Read the model definition and answer for the solid it produces. Units are mm, in the model's axes. A direction names the side the tool comes from. Coordinates: 2 decimals unless noted, no trailing zeros. Order: outer loops, then holes, each group sorted by start corner. A loop starts at its lowest first (then second) coordinate and runs counter-clockwise, first axis right, second up. Notation, with made-up numbers: (-29.75, 88) - (-14.75, 88) arc R8 ccw to (-14.75, 93) - close; hole circle Ø7 at (-9, 14). An arc over 180 degrees is marked (long way). Use one line per item in the form item = value. Start each with the question number.
from build123d import *

# Parameters (mm, degrees)
RESSALTO_EXTRUS_O1_DEPTH     = 181.5
CORTE_EXTRUS_O2_DEPTH        = 50
FURO_DE_DI_METRO_5_5_5_5_1_D = 5.5


with BuildPart() as part:
    # Esboço1 → Ressalto-extrusão1 (new, symmetric)
    with BuildSketch(Plane.XY):
        Polygon((-12.7, 0), (12.7, 0), (12.7, -2), (1, -2), (1, -25.4), (-1, -25.4), (-1, -2), (-12.7, -2), align=None)
    extrude(amount=RESSALTO_EXTRUS_O1_DEPTH, both=True)

    # Esboço3 → Corte-extrusão2 (cut, symmetric)
    with BuildSketch(Plane(origin=(0, 0, 0), x_dir=(0, 0, -1), z_dir=(1, 0, 0))):
        Polygon((-177.5, -4), (-168, -4), (-168, -2), (-181.5, -2), (-181.5, -25.4), (-177.5, -25.4), align=None)
        Polygon((181.5, -25.4), (177.5, -25.4), (177.5, -4), (168, -4), (168, -2), (181.5, -2), align=None)
    extrude(amount=CORTE_EXTRUS_O2_DEPTH, both=True, mode=Mode.SUBTRACT)

    # Furo de diâmetro Ø5.5 (5.5)1 (through all)
    with Locations(Plane(origin=(0, 0, 0), x_dir=(1, 0, 0), z_dir=(0, 1, 0))):
        with Locations((5.2, -174), (-5.2, -174), (-5.2, 174), (5.2, 174)):
            Hole(FURO_DE_DI_METRO_5_5_5_5_1_D / 2)


solid = part.part
Q1. Given P1, Ø6, axis at x = 6, y = -10.5, coming from the -Z side; P2, Ø10, axis at x = 2, z = -4.5, coming from the -Y side; P3, Ø3, axis at x = -5, z = 38, coming from the -Y side; P4, Ø1.6, axis at x = 0.5, y = -3.5, coming from the +Z side, each flat-ended and moving along its own axis, determine where each tip first touches the part or whether it passes through.
Q2. For a pull along Z with two mould halves and no side action, classify faces 1 (the cylindrical face through (-4.604, -1.014, 176.685)), 2 (the flat face through (-1, -14, 2)) as +Z half, -Z half, draft (parallel to the pull), parting line (faces both ways), or undercut.
Q3. Consider probe 1 along Z at (x, y) = (5.2, -1.3); probe 2 along X at (y, z) = (-0.9, -174); probe 3 along X at (y, z) = (-3, -18). Determine where each line is inside the solid, lowest interval first.
Q4. A cutting plane is placed at A-A (z = 92). Give the vertices of the cut face in (x, y), then the cut area to 3 significant figures.
Q5. Which of the six approach directions +Z, -Z, +X, -X, +Y, -Y give full straight-line access (tool end or side, diameter ignored) to faces 3 (the cylindrical face through (5.796, -1.014, -171.315)), 4 (the flat face through (1, -14, 2))?
Q6. A cutting plane is placed at B-B (y = -21.75). Give the vertices of the cut face in (x, z).
Result sheet:
q1.P1 = through
q1.P2 = -25.4
q1.P3 = -2
q1.P4 = 177.5
q2.face_1 = undercut
q2.face_2 = draft
q3.probe_1 = -181.5 to -176.75, -171.25 to 171.25, 176.75 to 181.5
q3.probe_2 = -12.7 to -7.95, -2.45 to 2.45, 7.95 to 12.7
q3.probe_3 = -1 to 1
q4.outline = (-12.7, -2) - (-1, -2) - (-1, -25.4) - (1, -25.4) - (1, -2) - (12.7, -2) - (12.7, 0) - (-12.7, 0) - close
q4.area = 97.6 mm^2
q5.face_3 = +Y, -Y
q5.face_4 = +Z, -Z, +X, -Y
q6.outline = (-1, -177.5) - (1, -177.5) - (1, 177.5) - (-1, 177.5) - close
